from build123d import *

# Parameters (mm, degrees)
BOSS_EXTRUDE1_DEPTH = 38
SKETCH2_W           = 20
SKETCH2_H           = 11
CUT_EXTRUDE1_DEPTH  = 145.390096613
CIRPATTERN1_COUNT   = 26


with BuildPart() as part:
    # Sketch1 → Boss-Extrude1 (new body)
    with BuildSketch(Plane(origin=(0, 0, 0), x_dir=(1, 0, 0), z_dir=(0, 1, 0))):
        with BuildLine():
            ThreePointArc((76.973491541, -61.46), (79.050100656, -58.765054125), (81.032400927, -56))
            Line((81.032400927, -56), (77.974354758, -56))
            ThreePointArc((77.974354758, -56), (75.90994771, -58.76801714), (73.747328087, -61.46))
            Line((73.747328087, -61.46), (76.973491541, -61.46))
        make_face()
        with BuildLine():
            ThreePointArc((73.747328087, -61.46), (75.90994771, -58.76801714), (77.974354758, -56))
            Line((77.974354758, -56), (-77.974354758, -56))
            ThreePointArc((-77.974354758, -56), (-75.90994771, -58.76801714), (-73.747328087, -61.46))
            Line((-73.747328087, -61.46), (73.747328087, -61.46))
        make_face()
        with BuildLine():
            ThreePointArc((-73.747328087, -61.46), (-75.90994771, -58.76801714), (-77.974354758, -56))
            Line((-77.974354758, -56), (-81.032400927, -56))
            ThreePointArc((-81.032400927, -56), (-79.050100656, -58.765054125), (-76.973491541, -61.46))
            Line((-76.973491541, -61.46), (-73.747328087, -61.46))
        make_face()
        with BuildLine():
            Line((77.974354758, -56), (81.032400927, -56))
            ThreePointArc((81.032400927, -56), (94.031753922, -29.330517458), (98.5, 0))
            ThreePointArc((98.5, 0), (-29.330517458, 94.031753922), (-81.032400927, -56))
            Line((-81.032400927, -56), (-77.974354758, -56))
            ThreePointArc((-77.974354758, -56), (-29.414808713, 91.382542252), (96, 0))
            ThreePointArc((96, 0), (91.382542252, -29.414808713), (77.974354758, -56))
        make_face()
        with BuildLine():
            ThreePointArc((-76.973491541, -61.46), (0, -98.5), (76.973491541, -61.46))
            Line((76.973491541, -61.46), (73.747328087, -61.46))
            ThreePointArc((73.747328087, -61.46), (0, -96), (-73.747328087, -61.46))
            Line((-73.747328087, -61.46), (-76.973491541, -61.46))
        make_face()
    extrude(amount=BOSS_EXTRUDE1_DEPTH)

    # Sketch2 → Cut-Extrude1 (cut, through all)
    with BuildSketch(Plane(origin=(0, 0, 0), x_dir=(0, 0, -1), z_dir=(1, 0, 0))):
        with Locations((0, 19.5)):
            Rectangle(SKETCH2_W, SKETCH2_H)
    cut_extrude1 = extrude(amount=-CUT_EXTRUDE1_DEPTH, mode=Mode.SUBTRACT)

    # CirPattern1: Cut-Extrude1 ×26 about axis
    cirpattern1_axis = Axis((0, 0, 0), (0, 1, 0))
    for i in range(1, CIRPATTERN1_COUNT):
        add(cut_extrude1.rotate(cirpattern1_axis, i * 360 / CIRPATTERN1_COUNT), mode=Mode.SUBTRACT)


solid = part.part
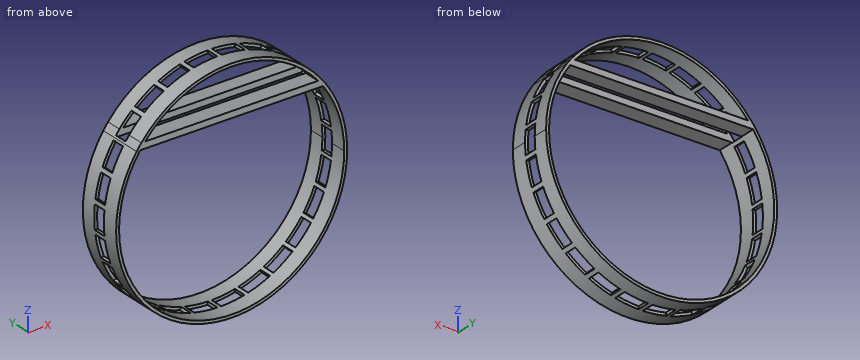
Could you check a few things on this model? Use its own coordinates, in mm. Give positions to 0.01 mm unless a question says otherwise; leave off trailing zeros. Order: outer loops, then holes, each group sorted by start corner. A loop starts at its lowest first (then second) coordinate and runs counter-clockwise, first axis right, second up.
1. Suppose I cut it at C-C (x = 32). List the corners of the cut face in (y, z) for me.
2. Will these pins go through, and if not, where does the flat tip stop? P1, Ø6, axis at y = 11, z = 75, coming from the -X side; P2, Ø1.5, axis at y = 34, z = -45.5, coming from the +X side; P3, Ø12, axis at x = 66, y = 19.5, coming from the +Z side; P4, Ø4, axis at x = -51, z = 78.5, coming from the +Y side.
3. Suppose I cut it at B-B (z = -65). List the corners of the cut face in (x, y) for me, plus the area to 3 significant figures.
4. Suppose I cut it at A-A (y = 34). List the corners of the cut face in (x, z) for me, plus the area to 3 significant figures.
5. Suppose I cut it at D-D (y = 17). Give the number of separate pieces and of enclosed holes in the cut face, plus the area to 3 significant figures.
6. I need wall thicknesses on L1, parallel to Z at x = 0, y = 27; L2, parallel to X at y = 11, z = 1; L3, parallel to Z at x = 0, y = 21. Which ranges of each line are inside material? Lowest first, please.
Solved:
1. outline: (0, -93.16) - (14, -93.16) - (14, -90.51) - (0, -90.51) - close; (0, 56) - (14, 56) - (14, 61.46) - (0, 61.46) - close; (0, 90.51) - (14, 90.51) - (14, 93.16) - (0, 93.16) - close; (25, -93.16) - (38, -93.16) - (38, -90.51) - (25, -90.51) - close; (25, 56) - (38, 56) - (38, 61.46) - (25, 61.46) - close; (25, 90.51) - (38, 90.51) - (38, 93.16) - (25, 93.16) - close
2. P1: stops at x = -67.22
2. P2: stops at x = 87.75
2. P3: stops at z = 75.21
2. P4: passes through
3. outline: (-74.01, 0) - (-70.65, 0) - (-70.65, 14) - (-74.01, 14) - close; (-74.01, 25) - (-70.65, 25) - (-70.65, 38) - (-74.01, 38) - close; (70.65, 0) - (74.01, 0) - (74.01, 14) - (70.65, 14) - close; (70.65, 25) - (74.01, 25) - (74.01, 38) - (70.65, 38) - close
3. area: 182 mm2
4. outline: circle Ø197 at (0, 0); hole (-77.97, 56) arc R96 ccw (long way) to (77.97, 56) - close; hole (-73.75, 61.46) - (73.75, 61.46) arc R96 ccw to start
4. area: 2,360 mm2
5. separate pieces: 26
5. enclosed holes: 0
5. area: 225 mm2
6. L1: z = -98.5 to -96, 56 to 61.46, 96 to 98.5
6. L2: x = -98.49 to -95.99, 95.99 to 98.49
6. L3: z = -98.5 to -96, 96 to 98.5
